Answer from the drawing. Dimensions are ordinates in mm from the lowest x, y and z of the part. Coordinates: 2 decimals unless noted, no trailing zeros. Write each loop counter-clockwise with the first axis right and the second up, starting at its lowest first coordinate (ties: lowest second). Pieces come first, ordered by that corner, then holes. Notation, with made-up numbers: M 44,21 L 91,21 A19 ccw 91,58 Z; hole C 52.5,-27 d5. An arc over 180 degrees is marked long. Put each result on its own line as item: value. Start each with the question number.
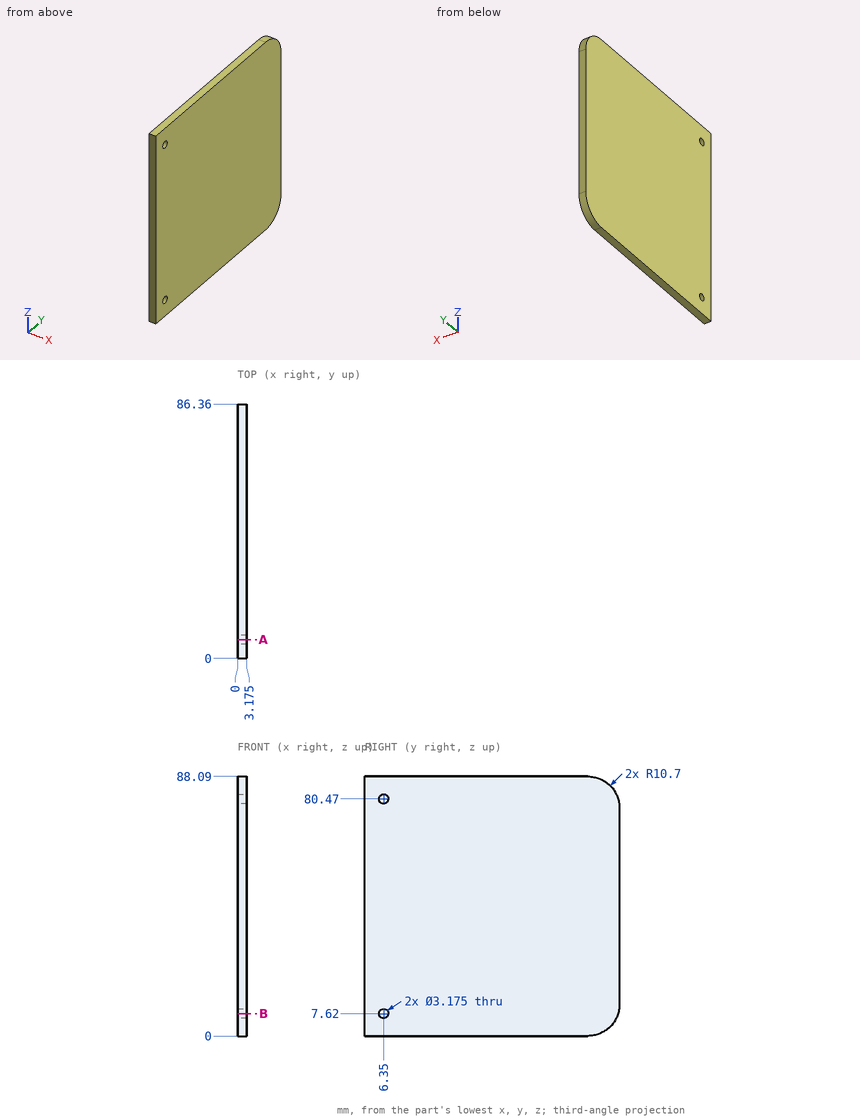
1) A cutting plane is placed at B-B on z = 7.62. Write down the section's boundary in (x, y) (1 decimal), then the cut area to 3 significant figures.
2) A cutting plane is placed at A-A on y = 6.35. Write down the section's boundary in (x, z) (1 decimal).
3) Given pin 1 Ø5 at (y, z) = (6.35, 7.62) entering from +X (3 decimals), flat-ended and moving along its own axis, determine where the tip first touches the part or whether it passes through.
4) Straight lines are drawn through the part: probe 1 along Y at (x, z) = (0.85, 7.62); probe 2 along Y at (x, z) = (1, 8); probe 3 along Y at (x, z) = (0.25, 10.5). For each, find the intervals that lie inside material, in ascending order.
Answers follow:
1. outline: M 0,0 L 3.2,0 L 3.2,4.8 L 0,4.8 Z; M 0,7.9 L 3.2,7.9 L 3.2,85.9 L 0,85.9 Z
1. area: 263 mm²
2. outline: M 0,0 L 3.2,0 L 3.2,6 L 0,6 Z; M 0,9.2 L 3.2,9.2 L 3.2,78.9 L 0,78.9 Z; M 0,82.1 L 3.2,82.1 L 3.2,88.1 L 0,88.1 Z
3. pin 1: stops at x = 3.175
4. probe 1: y = 0 to 4.76, 7.94 to 85.91
4. probe 2: y = 0 to 4.81, 7.89 to 86.01
4. probe 3: y = 0 to 86.36
